from build123d import *

# Parameters (mm, degrees)
SKETCH_1_W                      = 25
SKETCH_1_H                      = 50
EXTRUDE_1_DEPTH                 = 3
EXTRUDE_2_DEPTH                 = 25
CUT_EXTRUDE_1_REACH             = 5
SKETCH_2_R                      = 2.5
SKETCH_2_R_2                    = 4
SKETCH_2_R_3                    = 2
CUT_EXTRUDE_1_DIRECTION_2_REACH = 30


with BuildPart() as part:
    # 草图1 → 凸台-拉伸1 (new body)
    with BuildSketch(Plane.XY):
        with Locations((12.5, 25)):
            Rectangle(SKETCH_1_W, SKETCH_1_H)
    extrude(amount=EXTRUDE_1_DEPTH)

    # 草图4 → 凸台-拉伸2 (add)
    with BuildSketch(Plane.ZY):
        Polygon((-23, -3), (-23, 20.018133071), (-28, 20.018133071), (-28, 50), (-25, 50), (-25, 23.018133071), (-20, 23.018133071), (-20, 0), (3, 0), (3, -3), align=None)
    extrude(amount=-EXTRUDE_2_DEPTH)

    # 草图2 → 切除-拉伸1 (cut, up to next)
    with BuildSketch(Plane(origin=(0, 0, 0), x_dir=(-1, 0, 0), z_dir=(0, 0, -1)), mode=Mode.PRIVATE) as cut_extrude_1_sk1:
        with Locations((-18.5, 10)):
            Circle(SKETCH_2_R)
    cut_extrude_1_tool1 = extrude(cut_extrude_1_sk1.sketch, amount=-CUT_EXTRUDE_1_REACH, mode=Mode.PRIVATE) & part.part
    add(cut_extrude_1_tool1.solids().sort_by_distance((18.5, 10, 0))[0], mode=Mode.SUBTRACT)
    # 草图2 → 切除-拉伸1 (cut, up to next)
    with BuildSketch(Plane(origin=(0, 0, 0), x_dir=(-1, 0, 0), z_dir=(0, 0, -1)), mode=Mode.PRIVATE) as cut_extrude_1_sk2:
        with Locations((-6.5, 10)):
            Circle(SKETCH_2_R)
    cut_extrude_1_tool2 = extrude(cut_extrude_1_sk2.sketch, amount=-CUT_EXTRUDE_1_REACH, mode=Mode.PRIVATE) & part.part
    add(cut_extrude_1_tool2.solids().sort_by_distance((6.5, 10, 0))[0], mode=Mode.SUBTRACT)
    # 草图2 → 切除-拉伸1 (cut, up to next)
    with BuildSketch(Plane(origin=(0, 0, 0), x_dir=(-1, 0, 0), z_dir=(0, 0, -1)), mode=Mode.PRIVATE) as cut_extrude_1_sk3:
        with Locations((-12.5, 40)):
            Circle(SKETCH_2_R_2)
    cut_extrude_1_tool3 = extrude(cut_extrude_1_sk3.sketch, amount=-CUT_EXTRUDE_1_REACH, mode=Mode.PRIVATE) & part.part
    add(cut_extrude_1_tool3.solids().sort_by_distance((12.5, 40, 0))[0], mode=Mode.SUBTRACT)
    # 草图2 → 切除-拉伸1 (cut, up to next)
    with BuildSketch(Plane(origin=(0, 0, 0), x_dir=(-1, 0, 0), z_dir=(0, 0, -1)), mode=Mode.PRIVATE) as cut_extrude_1_sk4:
        with Locations((-6.5, 46)):
            Circle(SKETCH_2_R_3)
    cut_extrude_1_tool4 = extrude(cut_extrude_1_sk4.sketch, amount=-CUT_EXTRUDE_1_REACH, mode=Mode.PRIVATE) & part.part
    add(cut_extrude_1_tool4.solids().sort_by_distance((6.5, 46, 0))[0], mode=Mode.SUBTRACT)
    # 草图2 → 切除-拉伸1 (cut, up to next)
    with BuildSketch(Plane(origin=(0, 0, 0), x_dir=(-1, 0, 0), z_dir=(0, 0, -1)), mode=Mode.PRIVATE) as cut_extrude_1_sk5:
        with Locations((-6.5, 34)):
            Circle(SKETCH_2_R_3)
    cut_extrude_1_tool5 = extrude(cut_extrude_1_sk5.sketch, amount=-CUT_EXTRUDE_1_REACH, mode=Mode.PRIVATE) & part.part
    add(cut_extrude_1_tool5.solids().sort_by_distance((6.5, 34, 0))[0], mode=Mode.SUBTRACT)
    # 草图2 → 切除-拉伸1 (cut, up to next)
    with BuildSketch(Plane(origin=(0, 0, 0), x_dir=(-1, 0, 0), z_dir=(0, 0, -1)), mode=Mode.PRIVATE) as cut_extrude_1_sk6:
        with Locations((-18.5, 34)):
            Circle(SKETCH_2_R_3)
    cut_extrude_1_tool6 = extrude(cut_extrude_1_sk6.sketch, amount=-CUT_EXTRUDE_1_REACH, mode=Mode.PRIVATE) & part.part
    add(cut_extrude_1_tool6.solids().sort_by_distance((18.5, 34, 0))[0], mode=Mode.SUBTRACT)
    # 草图2 → 切除-拉伸1 (cut, up to next)
    with BuildSketch(Plane(origin=(0, 0, 0), x_dir=(-1, 0, 0), z_dir=(0, 0, -1)), mode=Mode.PRIVATE) as cut_extrude_1_sk7:
        with Locations((-18.5, 46)):
            Circle(SKETCH_2_R_3)
    cut_extrude_1_tool7 = extrude(cut_extrude_1_sk7.sketch, amount=-CUT_EXTRUDE_1_REACH, mode=Mode.PRIVATE) & part.part
    add(cut_extrude_1_tool7.solids().sort_by_distance((18.5, 46, 0))[0], mode=Mode.SUBTRACT)

    # 草图2 → 切除-拉伸1 direction 2 (cut, up to next)
    with BuildSketch(Plane(origin=(0, 0, 0), x_dir=(-1, 0, 0), z_dir=(0, 0, -1)), mode=Mode.PRIVATE) as cut_extrude_1_direction_2_sk1:
        with Locations((-18.5, 10)):
            Circle(SKETCH_2_R)
    cut_extrude_1_direction_2_tool1 = extrude(cut_extrude_1_direction_2_sk1.sketch, amount=CUT_EXTRUDE_1_DIRECTION_2_REACH, mode=Mode.PRIVATE) & part.part
    add(cut_extrude_1_direction_2_tool1.solids().sort_by_distance((18.5, 10, 0))[0], mode=Mode.SUBTRACT)
    # 草图2 → 切除-拉伸1 direction 2 (cut, up to next)
    with BuildSketch(Plane(origin=(0, 0, 0), x_dir=(-1, 0, 0), z_dir=(0, 0, -1)), mode=Mode.PRIVATE) as cut_extrude_1_direction_2_sk2:
        with Locations((-6.5, 10)):
            Circle(SKETCH_2_R)
    cut_extrude_1_direction_2_tool2 = extrude(cut_extrude_1_direction_2_sk2.sketch, amount=CUT_EXTRUDE_1_DIRECTION_2_REACH, mode=Mode.PRIVATE) & part.part
    add(cut_extrude_1_direction_2_tool2.solids().sort_by_distance((6.5, 10, 0))[0], mode=Mode.SUBTRACT)
    # 草图2 → 切除-拉伸1 direction 2 (cut, up to next)
    with BuildSketch(Plane(origin=(0, 0, 0), x_dir=(-1, 0, 0), z_dir=(0, 0, -1)), mode=Mode.PRIVATE) as cut_extrude_1_direction_2_sk3:
        with Locations((-12.5, 40)):
            Circle(SKETCH_2_R_2)
    cut_extrude_1_direction_2_tool3 = extrude(cut_extrude_1_direction_2_sk3.sketch, amount=CUT_EXTRUDE_1_DIRECTION_2_REACH, mode=Mode.PRIVATE) & part.part
    add(cut_extrude_1_direction_2_tool3.solids().sort_by_distance((12.5, 40, 0))[0], mode=Mode.SUBTRACT)
    # 草图2 → 切除-拉伸1 direction 2 (cut, up to next)
    with BuildSketch(Plane(origin=(0, 0, 0), x_dir=(-1, 0, 0), z_dir=(0, 0, -1)), mode=Mode.PRIVATE) as cut_extrude_1_direction_2_sk4:
        with Locations((-6.5, 46)):
            Circle(SKETCH_2_R_3)
    cut_extrude_1_direction_2_tool4 = extrude(cut_extrude_1_direction_2_sk4.sketch, amount=CUT_EXTRUDE_1_DIRECTION_2_REACH, mode=Mode.PRIVATE) & part.part
    add(cut_extrude_1_direction_2_tool4.solids().sort_by_distance((6.5, 46, 0))[0], mode=Mode.SUBTRACT)
    # 草图2 → 切除-拉伸1 direction 2 (cut, up to next)
    with BuildSketch(Plane(origin=(0, 0, 0), x_dir=(-1, 0, 0), z_dir=(0, 0, -1)), mode=Mode.PRIVATE) as cut_extrude_1_direction_2_sk5:
        with Locations((-6.5, 34)):
            Circle(SKETCH_2_R_3)
    cut_extrude_1_direction_2_tool5 = extrude(cut_extrude_1_direction_2_sk5.sketch, amount=CUT_EXTRUDE_1_DIRECTION_2_REACH, mode=Mode.PRIVATE) & part.part
    add(cut_extrude_1_direction_2_tool5.solids().sort_by_distance((6.5, 34, 0))[0], mode=Mode.SUBTRACT)
    # 草图2 → 切除-拉伸1 direction 2 (cut, up to next)
    with BuildSketch(Plane(origin=(0, 0, 0), x_dir=(-1, 0, 0), z_dir=(0, 0, -1)), mode=Mode.PRIVATE) as cut_extrude_1_direction_2_sk6:
        with Locations((-18.5, 34)):
            Circle(SKETCH_2_R_3)
    cut_extrude_1_direction_2_tool6 = extrude(cut_extrude_1_direction_2_sk6.sketch, amount=CUT_EXTRUDE_1_DIRECTION_2_REACH, mode=Mode.PRIVATE) & part.part
    add(cut_extrude_1_direction_2_tool6.solids().sort_by_distance((18.5, 34, 0))[0], mode=Mode.SUBTRACT)
    # 草图2 → 切除-拉伸1 direction 2 (cut, up to next)
    with BuildSketch(Plane(origin=(0, 0, 0), x_dir=(-1, 0, 0), z_dir=(0, 0, -1)), mode=Mode.PRIVATE) as cut_extrude_1_direction_2_sk7:
        with Locations((-18.5, 46)):
            Circle(SKETCH_2_R_3)
    cut_extrude_1_direction_2_tool7 = extrude(cut_extrude_1_direction_2_sk7.sketch, amount=CUT_EXTRUDE_1_DIRECTION_2_REACH, mode=Mode.PRIVATE) & part.part
    add(cut_extrude_1_direction_2_tool7.solids().sort_by_distance((18.5, 46, 0))[0], mode=Mode.SUBTRACT)


solid = part.part
The model under review builds one solid part; all positions refer to its coordinate system, in mm. A direction names the side the tool comes from. Give positions to 0.01 mm unless a question says otherwise; leave off trailing zeros. Order: outer loops, then holes, each group sorted by start corner. A loop starts at its lowest first (then second) coordinate and runs counter-clockwise, first axis right, second up. Notation, with made-up numbers: M 10.5,-7.75 L 34.5,-7.75 A18 ccw 34.5,-1.75 Z; hole C -13.75,-16 d2. An arc over 180 degrees is marked long. One line per question, with ' | ' between items. Start each with the question number.
1) Consider section C-C, the plane z = -26. Give the boundary of the cut face in (x, y).
2) For faces 4 (the face through (12, 8, -23)), 5 (the face through (12, 25, 0)), 6 (the face through (18.934, 32.048, 1.479)), list the 3-axis set-ups (+Z, -Z, +X, -X, +Y, -Y) from which the entire face can be reached by the end or side of a thin tool; tool diameter is ignored.
3) Consider section D-D, the plane y = 10. Give the boundary of the cut face in (x, z), then the cut area to 3 significant figures.
4) Mouldability with a two-part tool opening along X and no side actions: class faces 1 (the face through (12, 35, -28)), 2 (the face through (13.021, 43.966, -26.479)), 3 (the face through (0, 21.7, -20.5)) as pulls with the +X half, pulls with the -X half, needs draft (parallel to the pull), parting line crosses it, or undercut.
5) Consider section A-A, the plane y = 40. Give the boundary of the cut face in (x, z).
6) Consider section B-B, the plane x = 12.5. Give the boundary of the cut face in (y, z).
7) Wall thickness on L1, parallel to Y at x = 6.5, z = -26.65; L2, parallel to X at y = 34, z = -26; L3, parallel to Z at x = 1.5, y = 40: over which ranges is each line inside the solid? List them lowest first. Write a range as from..to.
Found:
1) outline: M 0,20.02 L 25,20.02 L 25,50 L 0,50 Z; hole C 6.5,34 d4; hole C 6.5,46 d4; hole C 12.5,40 d8; hole C 18.5,34 d4; hole C 18.5,46 d4
2) face 4: -Z, +X, -X, -Y | face 5: +X, -X, +Y | face 6: +Z, -Z
3) outline: M 0,-23 L 4,-23 L 4,-20 L 0,-20 Z; M 0,0 L 4,0 L 4,3 L 0,3 Z; M 9,-23 L 16,-23 L 16,-20 L 9,-20 Z; M 9,0 L 16,0 L 16,3 L 9,3 Z; M 21,-23 L 25,-23 L 25,-20 L 21,-20 Z; M 21,0 L 25,0 L 25,3 L 21,3 Z | area: 90.0 mm²
4) face 1: needs draft | face 2: undercut | face 3: pulls with the -X half
5) outline: M 0,-28 L 8.5,-28 L 8.5,-25 L 0,-25 Z; M 0,0 L 8.5,0 L 8.5,3 L 0,3 Z; M 16.5,-28 L 25,-28 L 25,-25 L 16.5,-25 Z; M 16.5,0 L 25,0 L 25,3 L 16.5,3 Z
6) outline: M -3,-23 L 20.02,-23 L 20.02,-28 L 36,-28 L 36,-25 L 23.02,-25 L 23.02,-20 L 0,-20 L 0,0 L 36,0 L 36,3 L -3,3 Z; M 44,-28 L 50,-28 L 50,-25 L 44,-25 Z; M 44,0 L 50,0 L 50,3 L 44,3 Z
7) L1: y = 20.02..32, 36..44, 48..50 | L2: x = 0..4.5, 8.5..16.5, 20.5..25 | L3: z = -28..-25, 0..3
